```python
from build123d import *

# Parameters (mm, degrees)
F0_R      = 25.4
F1_DEPTH  = 6.35
F2_R      = 22.225
F3_DEPTH  = 12.7
F4_R      = 25.4
F5_DEPTH  = 6.35
F6_R      = 1.5875
F6_R_2    = 6.35
F7_DEPTH  = 89
F9_D      = 12.7
F11_D     = 3.175
F11_DEPTH = 6.35
F11_TIP   = 0.9538662327
F13_D     = 3.175
F13_DEPTH = 6.35
F13_TIP   = 0.9538662327
F15_D     = 3.175
F15_DEPTH = 6.35
F15_TIP   = 0.9538662327
F17_D     = 3.175
F17_DEPTH = 6.35
F17_TIP   = 0.9538662327


# Not quite as in the source:
# - an extrude ends at something that could not be found from the text; its depth is read off the source's solid


with BuildPart() as f1:
    # F0 (on Front) → F1 (new body)
    with BuildSketch(Plane.XZ):
        Circle(F0_R)
    extrude(amount=F1_DEPTH)

    # F2 (on face) → F3 (join)
    with BuildSketch(Plane.XZ.offset(6.35)):
        Circle(F2_R)
    extrude(amount=F3_DEPTH)

    # F4 (on face) → F5 (join)
    with BuildSketch(Plane.XZ.offset(19.05)):
        Circle(F4_R)
    extrude(amount=F5_DEPTH)

    # F6 (on face) → F7 (cut, through all)
    with BuildSketch(Plane.XZ.offset(25.4)):
        with Locations((0, -20.6375)):
            Circle(F6_R)
        with Locations((20.6375, 0)):
            Circle(F6_R)
        with Locations((0, 20.6375)):
            Circle(F6_R)
        with Locations((-20.6375, 0)):
            Circle(F6_R)
        Circle(F6_R_2)
    extrude(amount=F7_DEPTH, mode=Mode.SUBTRACT)

    # F9 (through all)
    with Locations(Plane.XZ.offset(25.4)):
        with Locations((0, 0)):
            Hole(F9_D / 2)

    # F11
    with Locations(Plane.XZ.offset(25.4)):
        with Locations((19.05, 0)):
            Hole(F11_D / 2, depth=F11_DEPTH)
            with Locations((0, 0, -(F11_DEPTH + F11_TIP / 2))):  # 118° drill point
                Cone(0, F11_D / 2, F11_TIP, mode=Mode.SUBTRACT)

    # F13
    with Locations(Plane.XZ.offset(25.4)):
        with Locations((0, 19.05)):
            Hole(F13_D / 2, depth=F13_DEPTH)
            with Locations((0, 0, -(F13_DEPTH + F13_TIP / 2))):  # 118° drill point
                Cone(0, F13_D / 2, F13_TIP, mode=Mode.SUBTRACT)

    # F15
    with Locations(Plane.XZ.offset(25.4)):
        with Locations((-19.05, 0)):
            Hole(F15_D / 2, depth=F15_DEPTH)
            with Locations((0, 0, -(F15_DEPTH + F15_TIP / 2))):  # 118° drill point
                Cone(0, F15_D / 2, F15_TIP, mode=Mode.SUBTRACT)

    # F17
    with Locations(Plane.XZ.offset(25.4)):
        with Locations((1.4731416013, -19.0587695688)):
            Hole(F17_D / 2, depth=F17_DEPTH)
            with Locations((0, 0, -(F17_DEPTH + F17_TIP / 2))):  # 118° drill point
                Cone(0, F17_D / 2, F17_TIP, mode=Mode.SUBTRACT)


solid = f1.part
```
Build history of the part. All positions in model axes, mm. A direction names the side the tool comes from. Give positions to 0.01 mm unless a question says otherwise; leave off trailing zeros. Order: outer loops, then holes, each group sorted by start corner. A loop starts at its lowest first (then second) coordinate and runs counter-clockwise, first axis right, second up. Notation, with made-up numbers: M 25.25,41.25 L 80.25,41.25 A21 ccw 80.25,49.25 Z; hole C 40.5,52 d7. An arc over 180 degrees is marked long. Return JSON: item names as keys, results as strings.
Q1. Two-plate mould, pull along Z, no slides. Class faces 4 (the face through (-0.1, -6.35, -22.5)), 5 (the face through (20.636, -22.181, 0.07)), 6 (the face through (21.199, -12.611, 6.676)): pulls with the +Z half, pulls with the -Z half, needs draft (parallel to the pull), parting line crosses it, or undercut.
Answer list:
{"face 4": "needs draft", "face 5": "undercut", "face 6": "parting line crosses it"}
Q2. Wall check: probe 1 along Y at (x, z) = (7.5, -22.5); probe 2 along X at (y, z) = (-20.5, 19.05); probe 3 along Z at (x, y) = (-1, -4.75). Give the ranges that are in metal, low to high. Write a range as from..to.
Answer list:
{"probe 1": "y = -25.4..-19.05, -6.35..0", "probe 2": "x = -16.8..-1.59, 1.59..16.8", "probe 3": "z = -25.38..-6.27, 6.27..25.38"}
Q3. Band-saw the part on D-D (z = 9.5). Give the cut face in (x, y), then the cut area to 3 significant figures.
Answer list:
{"outline": "M -23.56,-25.4 L 23.56,-25.4 L 23.56,-19.05 L 20.09,-19.05 L 20.09,-6.35 L 23.56,-6.35 L 23.56,0 L -23.56,0 L -23.56,-6.35 L -20.09,-6.35 L -20.09,-19.05 L -23.56,-19.05 Z", "area": "1,110 mm^2"}
Q4. Band-saw the part on A-A (z = -2.5). Give the cut face in (x, y).
Answer list:
{"outline": "M -25.28,-25.4 L -5.84,-25.4 L -5.84,0 L -25.28,0 L -25.28,-6.35 L -22.08,-6.35 L -22.08,-19.05 L -25.28,-19.05 Z; M 5.84,-25.4 L 25.28,-25.4 L 25.28,-19.05 L 22.08,-19.05 L 22.08,-6.35 L 25.28,-6.35 L 25.28,0 L 5.84,0 Z"}
Q5. Band-saw the part on B-B (y = -1.75). Give the cut face in (x, z).
Answer list:
{"outline": "C 0,0 d50.8; hole C 0,0 d12.7"}
Q6. 3-axis set-ups, long thin cutter, end or side, ignore diameter. For faces 1 (the face through (-0.1, -19.05, -22.5)), 2 (the face through (0.34, -22.18, 17.5)), 3 (the face through (-5.506, -22.181, -24.796)): which of +Z, -Z, +X, -X, +Y, -Y reach the whole face in a straight line?
Answer list:
{"face 1": "none", "face 2": "-Y", "face 3": "+Y, -Y"}
Q7. Flat gauge pins, fed straight in: pin 1 (1.5 mm diameter, centred on x = -0.5, y = -22, fed in from -Z); pin 2 (10 mm diameter, centred on x = 0, z = 0, fed in from +Y); pin 3 (8 mm diameter, centred on x = 14.5, y = -16, fed in from -Z); pin 4 (3 mm diameter, centred on x = -4.5, y = -13, fed in from -Z). Where does each tip first touch, or does it go through?
Answer list:
{"pin 1": "stops at z = -25.4", "pin 2": "passes through", "pin 3": "stops at z = -22.43", "pin 4": "stops at z = -22.02"}
Q8. Band-saw the part on C-C (x = -14). Give the cut face in (y, z), then the cut area to 3 significant figures.
Answer list:
{"outline": "M -25.4,-21.19 L -19.05,-21.19 L -19.05,-17.26 L -6.35,-17.26 L -6.35,-21.19 L 0,-21.19 L 0,21.19 L -6.35,21.19 L -6.35,17.26 L -19.05,17.26 L -19.05,21.19 L -25.4,21.19 Z", "area": "977 mm^2"}
